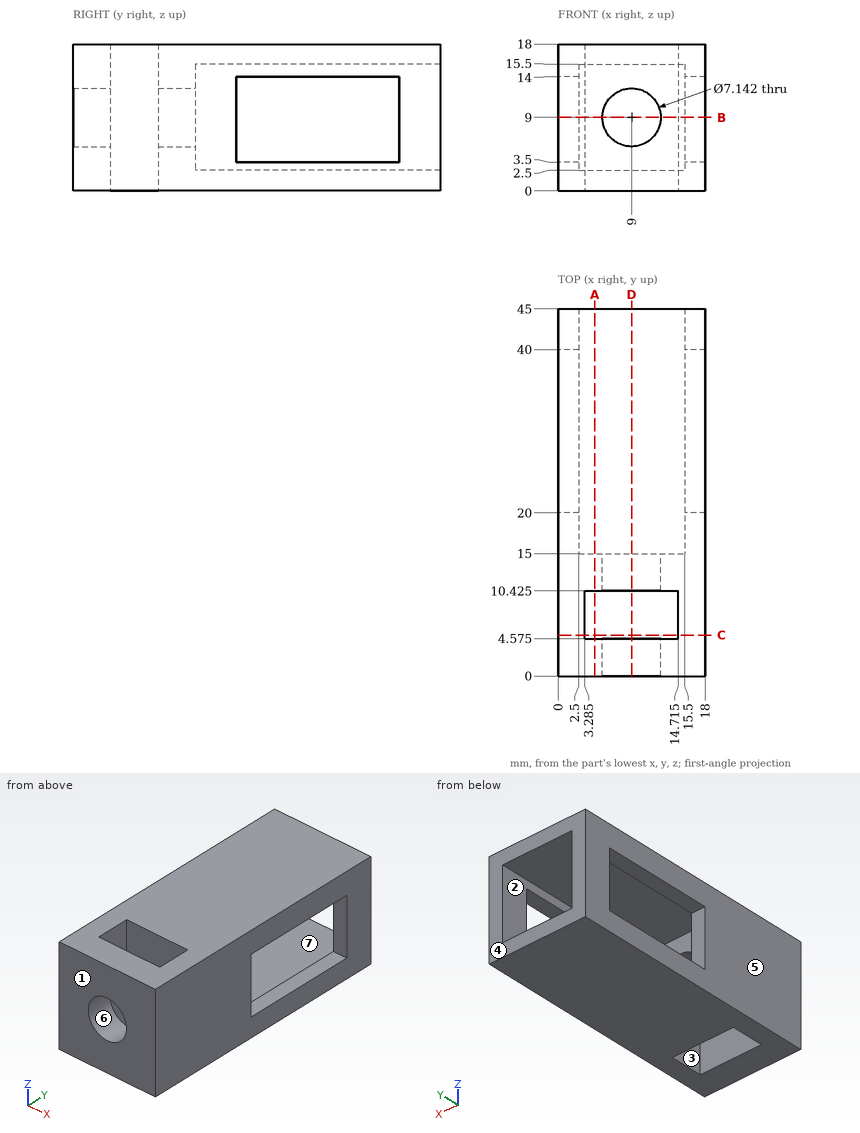
Source: three-view drawing plus pictorial views. Frame: mm from the lowest corner of the part. A direction names the side the tool comes from. Give positions to 0.01 mm unless a question says otherwise; leave off trailing zeros. Order: outer loops, then holes, each group sorted by start corner. A loop starts at its lowest first (then second) coordinate and runs counter-clockwise, first axis right, second up. Notation, with made-up numbers: M -34,64.25 L 22,64.25 A25 ccw 22,91.25 Z; hole C -39.5,60 d4. An arc over 180 degrees is marked long. One line per question, with ' | ' between items. Start each with the question number.
1. Pull-direction query (X, two-part tool) for the marked faces 4, 5, 6 and 7; classes: released by +X, released by -X, zero draft, split by the parting line, or undercut.
2. Material intervals for probe 1 along Y at (x, z) = (3.5, 14.75) (1 decimal); probe 2 along Z at (x, y) = (9, 32); probe 3 along Y at (x, z) = (10.75, 1) (1 decimal), sorted ascending. Write a range as [from, to].
3. Access query for the marked faces 1, 2 and 3. Directions: +Z, -Z, +X, -X, +Y, -Y. A direction counts if a zero-diameter tool reaches every point of the face in a straight line with its end or side. Return the directions, or none.
4. Section query C-C (y = 5). Return the cut outline in (x, z) (1 decimal).
5. Section query D-D (x = 9). Return the cut outline in (y, z) (1 decimal).
6. Section query B-B (z = 9). Return the cut outline in (x, y) (1 decimal), and give its area (3 significant figures).
7. Section query A-A (x = 4.5). Return the cut outline in (y, z) (1 decimal).
8. First-contact query: pin 1 Ø5.5 at (x, z) = (7.5, 7.5) entering from +Y. Flat tip, straight axial feed; report the tip coordinate or a pass-through.
Here are the results:
1) face 4: zero draft | face 5: released by -X | face 6: undercut | face 7: undercut
2) probe 1: [0, 4.6], [10.4, 15] | probe 2: [0, 2.5], [15.5, 18] | probe 3: [0, 4.6], [10.4, 45]
3) face 1: +Z, -Z, +X, -X, -Y | face 2: +Y | face 3: +Z, -Z
4) outline: M 0,0 L 3.3,0 L 3.3,18 L 0,18 Z; M 14.7,0 L 18,0 L 18,18 L 14.7,18 Z
5) outline: M 0,0 L 4.6,0 L 4.6,5.4 L 0,5.4 Z; M 0,12.6 L 4.6,12.6 L 4.6,18 L 0,18 Z; M 10.4,0 L 45,0 L 45,2.5 L 15,2.5 L 15,5.4 L 10.4,5.4 Z; M 10.4,12.6 L 15,12.6 L 15,15.5 L 45,15.5 L 45,18 L 10.4,18 Z
6) outline: M 0,0 L 5.4,0 L 5.4,4.6 L 3.3,4.6 L 3.3,10.4 L 5.4,10.4 L 5.4,15 L 2.5,15 L 2.5,20 L 0,20 Z; M 0,40 L 2.5,40 L 2.5,45 L 0,45 Z; M 12.6,0 L 18,0 L 18,20 L 15.5,20 L 15.5,15 L 12.6,15 L 12.6,10.4 L 14.7,10.4 L 14.7,4.6 L 12.6,4.6 Z; M 15.5,40 L 18,40 L 18,45 L 15.5,45 Z | area: 188 mm²
7) outline: M 0,0 L 4.6,0 L 4.6,18 L 0,18 Z; M 10.4,0 L 45,0 L 45,2.5 L 15,2.5 L 15,15.5 L 45,15.5 L 45,18 L 10.4,18 Z
8) pin 1: y = 15
